Check sheet for the drawn part. Datum: minimum x, y, z corner. Units: mm. Round coordinates to 2 decimals unless told otherwise and drop trailing zeros. Order: outer loops, then holes, each group sorted by start corner. A loop starts at its lowest first (then second) coordinate and runs counter-clockwise, first axis right, second up. Notation, with made-up numbers: (-30, 13) -> (17, 13) arc R14 cw to (17, 34) -> close; hole circle Ø2 at (-38, 53.25). An arc over 180 degrees is marked (long way). Use CSV: the item, a comma, the result in double quotes.
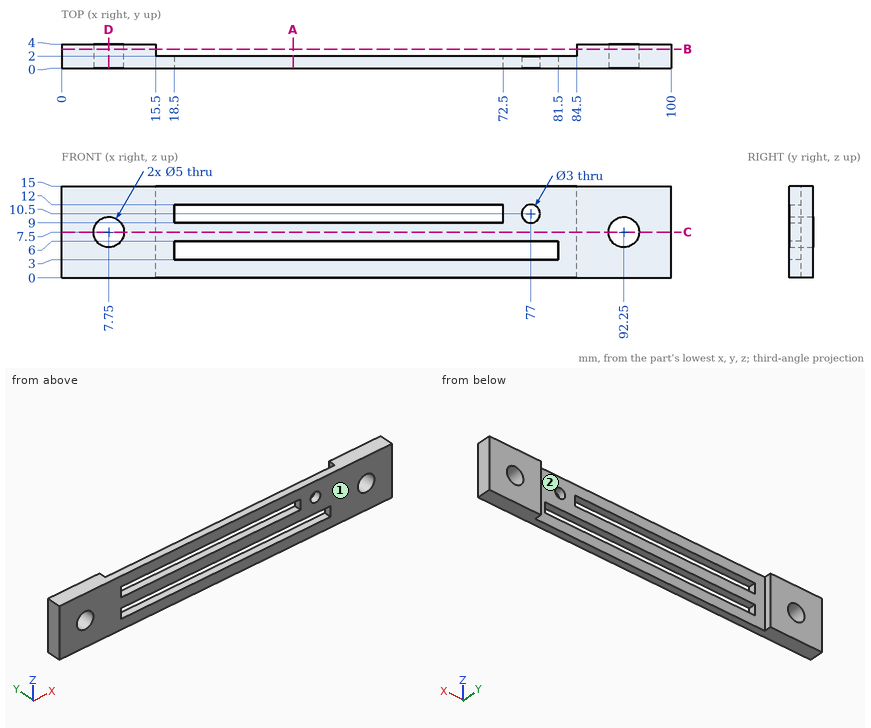
Q1. Sectioned sample at B-B, the plane y = 3.15. Enter the section's corners in (x, z), then the cut area to 3 significant figures.
Result sheet:
outline,"(0, 0) -> (15.5, 0) -> (15.5, 15) -> (0, 15) -> close; (84.5, 0) -> (100, 0) -> (100, 15) -> (84.5, 15) -> close; hole circle Ø5 at (7.75, 7.5); hole circle Ø5 at (92.25, 7.5)"
area,"426 mm^2"
Q2. Go/stop test with flat-tipped pins: pin 1 (1.5 mm diameter, centred on y = 3.5, z = 7, fed in from -X); pin 2 (4.5 mm diameter, centred on x = 92.25, z = 7.5, fed in from +Y); pin 3 (4 mm diameter, centred on x = 18, z = 4, fed in from +Y). Record where each tip stops, or that it passes through.
Result sheet:
pin 1,"stops at x = 0"
pin 2,"passes through"
pin 3,"stops at y = 2"
Q3. Sectioned sample at D-D, the plane x = 7.75. Enter the section's corners in (y, z), then the cut area to 3 significant figures.
Result sheet:
outline,"(0, 0) -> (4, 0) -> (4, 5) -> (0, 5) -> close; (0, 10) -> (4, 10) -> (4, 15) -> (0, 15) -> close"
area,"40.0 mm^2"
Q4. Sectioned sample at A-A, the plane x = 38. Enter the section's corners in (y, z), then the cut area to 3 significant figures.
Result sheet:
outline,"(0, 0) -> (2, 0) -> (2, 3) -> (0, 3) -> close; (0, 6) -> (2, 6) -> (2, 9) -> (0, 9) -> close; (0, 12) -> (2, 12) -> (2, 15) -> (0, 15) -> close"
area,"18.0 mm^2"
Q5. Sectioned sample at C-C, the plane z = 7.5. Enter the section's corners in (x, y).
Result sheet:
outline,"(0, 0) -> (5.25, 0) -> (5.25, 4) -> (0, 4) -> close; (10.25, 0) -> (89.75, 0) -> (89.75, 4) -> (84.5, 4) -> (84.5, 2) -> (15.5, 2) -> (15.5, 4) -> (10.25, 4) -> close; (94.75, 0) -> (100, 0) -> (100, 4) -> (94.75, 4) -> close"
Q6. Mould release check, pull along X, two halves, no side actions. Record for the marked faces 1 and 2: pulls with the +X half, pulls with the -X half, needs draft (parallel to the pull), parting line crosses it, or undercut.
Result sheet:
face 1,"needs draft"
face 2,"undercut"
Q7. Scan lines: L1, parallel to Z at x = 66, y = 0.8; L2, parallel to X at y = 3.75, z = 13; L3, parallel to Z at x = 7.75, y = 2.3. Record each from-to range of solid material in increasing order.
Result sheet:
L1,"z = 0 to 3, 6 to 9, 12 to 15"
L2,"x = 0 to 15.5, 84.5 to 100"
L3,"z = 0 to 5, 10 to 15"
